Could you check a few things on this model? Use its own coordinates, in mm. A direction names the side the tool comes from. Coordinates: 2 decimals unless noted, no trailing zeros. Order: outer loops, then holes, each group sorted by start corner. A loop starts at its lowest first (then second) coordinate and runs counter-clockwise, first axis right, second up. Notation, with made-up numbers: M 66.5,8 L 122.5,8 A13 cw 122.5,24 Z; hole C -33.75,-19 d4. An arc over 180 degrees is marked long. Put each result on its own line as item: value. Start each with the question number.
```python
from build123d import *

# Parameters (mm, degrees)
F1_DEPTH = 3.175
F3_DEPTH = 3.175
F4_W     = 3.175
F4_H     = 3.175
F5_DEPTH = 38.1


with BuildPart() as f1:
    # F0 (on Front) → F1 (new body)
    with BuildSketch(Plane.XZ):
        Polygon((41.275, -19.05), (41.275, 19.05), (-41.275, 19.05), (-41.275, -19.05), (-38.1, -19.05), (-38.1, -1.5875), (-14.0845158286, -1.5875), (-1.5875, -7.8360079143), (-1.5875, -19.05), (1.5875, -19.05), (1.5875, -7.8360079143), (14.0845158286, -1.5875), (38.1, -1.5875), (38.1, -19.05), align=None)
        Polygon((-38.1, 1.5875), (-38.1, 15.875), (-1.5875, 15.875), (-1.5875, 7.8360079143), (-14.0845158286, 1.5875), align=None, mode=Mode.SUBTRACT)
        Polygon((0, -5.08), (-10.16, 0), (0, 5.08), (10.16, 0), align=None, mode=Mode.SUBTRACT)
        Polygon((1.5875, 15.875), (38.1, 15.875), (38.1, 1.5875), (14.0845158286, 1.5875), (1.5875, 7.8360079143), align=None, mode=Mode.SUBTRACT)
    extrude(amount=F1_DEPTH)

    # F2 (on face) → F3 (join)
    with BuildSketch(Plane.XY.offset(19.05)):
        Polygon((-82.55, 39.7002), (-41.275, -3.175), (-41.275, 0), (-38.1, 0), (-79.375, 42.8752), (-79.375, 39.7002), align=None)
        Polygon((79.375, 42.8752), (38.1, 0), (41.275, 0), (41.275, -3.175), (82.55, 39.7002), (79.375, 39.7002), align=None)
    extrude(amount=-F3_DEPTH)

    # F4 (on face) → F5 (join)
    with BuildSketch(Plane.XY.offset(19.05)):
        with Locations((-80.9625, 41.2877)):
            Rectangle(F4_W, F4_H)
        with Locations((80.9625, 41.2877)):
            Rectangle(F4_W, F4_H)
    extrude(amount=-F5_DEPTH)


solid = f1.part
```
Item 1: If we section it at D-D on x = -6.5: Write out the boundary of the cut face in (y, z) (3 decimals), then the cut area to 3 significant figures.
Item 2: If we section it at C-C on y = 9: Write out the boundary of the cut face in (x, z) (3 decimals).
Item 3: If we section it at B-B on z = 12: State how many separate pieces and enclosed holes the cut face has, then the cut area to 3 significant figures.
Item 4: For pin 1 Ø1.6 at (y, z) = (-1.5, -8) entering from -X (3 decimals); pin 2 Ø19 at (x, z) = (20.5, 0.5) entering from +Y; pin 3 Ø1 at (x, y) = (-23, -2.5) entering from -Z, each with a flat end and sliding along its axis, tell me the tip position at first contact or that it passes through.
Item 5: For faces 4 (the flat face through (-81, 39.7, -1)), 5 (the flat face through (26, -2, -1.588)), 6 (the flat face through (-81, 41, -19.05)), 7 (the flat face through (5.151, -1.565, -2.504)), 8 (the flat face through (-81, 42.875, 0)), which set-ups out of +Z, -Z, +X, -X, +Y, -Y let a thin tool reach every point of the face, with its end or its side?
Item 6: I need wall thicknesses on probe 1 along X at (y, z) = (-0.5, -12) (1 decimal); probe 2 along Z at (x, y) = (-56, 17) (3 decimals); probe 3 along X at (y, z) = (18, 17.5). Which ranges of each line are inside material? Lowest first, please.
Item 7: If we mould it in two halves opening along X, with no side actions, what happens to faces 1 (the flat face through (40, -2, -19.05)), 2 (the flat face through (-82.55, 41, 0)), 3 (the flat face through (-26, -2, 1.588))? For each: released by +X, released by -X, zero draft, split by the parting line, or undercut.
Geometry check:
1. outline: M -3.175,-5.38 L 0,-5.38 L 0,-1.83 L -3.175,-1.83 Z; M -3.175,1.83 L 0,1.83 L 0,5.38 L -3.175,5.38 Z; M -3.175,15.875 L 0,15.875 L 0,19.05 L -3.175,19.05 Z
1. area: 32.6 mm²
2. outline: M -52.996,15.875 L -46.764,15.875 L -46.764,19.05 L -52.996,19.05 Z; M 46.764,15.875 L 52.996,15.875 L 52.996,19.05 L 46.764,19.05 Z
3. separate pieces: 5
3. enclosed holes: 0
3. area: 50.4 mm²
4. pin 1: stops at x = -41.275
4. pin 2: stops at y = 0
4. pin 3: stops at z = -1.59
5. face 4: -Z, +X, -X, -Y
5. face 5: -Z, +Y, -Y
5. face 6: -Z, +X, -X, +Y, -Y
5. face 7: +Y, -Y
5. face 8: +Z, -Z, +X, -X, +Y
6. probe 1: x = -41.3 to -38.1, -1.6 to 1.6, 38.1 to 41.3
6. probe 2: z = 15.875 to 19.05
6. probe 3: x = -61.66 to -55.43, 55.43 to 61.66
7. face 1: zero draft
7. face 2: released by -X
7. face 3: undercut
